Model file for the job. Use its own axes, mm. A direction names the side the tool comes from. Round coordinates to 2 decimals unless told otherwise and drop trailing zeros. Order: outer loops, then holes, each group sorted by start corner. A loop starts at its lowest first (then second) coordinate and runs counter-clockwise, first axis right, second up. Notation, with made-up numbers: (37, 87.25) - (88, 87.25) arc R24 ccw to (88, 123.25) - close; hole circle Ø3 at (2, 13). An arc over 180 degrees is marked (long way). Put each result on its own line as item: value. Start each with the question number.
Item 1: Mould opens along X. For faces 3 (the face through (-285, 10, 5)), 4 (the face through (285, 10, 2)), 5 (the face through (-4, 3, -5)) say: pulls with the +X half, pulls with the -X half, needs draft (parallel to the pull), parting line crosses it, or undercut.
Item 2: Saw through at A-A on x = -91. List the corners of the cut face in (y, z), plus the area to 3 significant figures.
Item 3: Saw through at B-B on z = 13. List the corners of the cut face in (x, y).
Item 4: Probe probe 1 along Y at (x, z) = (25, -1.85); probe 2 along Y at (x, z) = (-11, 15.5); probe 3 along Z at (x, y) = (-195, 5.25). List the from-to ranges inside material, lowest first.
Item 5: Which spindle directions (+Z, -Z, +X, -X, +Y, -Y) get a long thin tool onto all of the face, cutting with end or side? Do faces 1 (the face through (-4, 8, 10)), 2 (the face through (-4, 13, 8)). Say none if no direction does.
```python
from build123d import *

# Parameters (mm, degrees)
F0_W     = 570
F0_H     = 5
F1_DEPTH = 20
F0_R     = 3
F0_W_2   = 5.1
F0_H_2   = 10.1
F0_W_3   = 6
F0_H_3   = 2
F2_DEPTH = 5


with BuildPart() as f1:
    # F0 (on Top) → F1 (new body)
    with BuildSketch(Plane.XY):
        with Locations((0, 10.5)):
            Rectangle(F0_W, F0_H)
    extrude(amount=F1_DEPTH)

    # F0 (on Top) → F2 (join)
    with BuildSketch(Plane.XY):
        with BuildLine():
            ThreePointArc((-285, -5), (-284.12132, -7.12132), (-282, -8))
            Line((-282, -8), (282, -8))
            ThreePointArc((282, -8), (284.12132, -7.12132), (285, -5))
            Line((285, -5), (285, 8))
            Line((285, 8), (-285, 8))
            Line((-285, 8), (-285, -5))
        make_face()
        with Locations((-275, 0)):
            Circle(F0_R, mode=Mode.SUBTRACT)
        with Locations((-220, 0)):
            Circle(F0_R, mode=Mode.SUBTRACT)
        with Locations((-80, 0)):
            Circle(F0_R, mode=Mode.SUBTRACT)
        with Locations((-25, 0)):
            Circle(F0_R, mode=Mode.SUBTRACT)
        Rectangle(F0_W_2, F0_H_2, mode=Mode.SUBTRACT)
        with Locations((25, 0)):
            Circle(F0_R, mode=Mode.SUBTRACT)
        with Locations((80, 0)):
            Circle(F0_R, mode=Mode.SUBTRACT)
        with Locations((220, 0)):
            Circle(F0_R, mode=Mode.SUBTRACT)
        with Locations((275, 0)):
            Circle(F0_R, mode=Mode.SUBTRACT)
        with Locations((-265, 6)):
            Rectangle(F0_W_3, F0_H_3, mode=Mode.SUBTRACT)
        with Locations((-210, 6)):
            Rectangle(F0_W_3, F0_H_3, mode=Mode.SUBTRACT)
        with Locations((-70, 6)):
            Rectangle(F0_W_3, F0_H_3, mode=Mode.SUBTRACT)
        with Locations((-35, 6)):
            Rectangle(F0_W_3, F0_H_3, mode=Mode.SUBTRACT)
        with Locations((35, 6)):
            Rectangle(F0_W_3, F0_H_3, mode=Mode.SUBTRACT)
        with Locations((70, 6)):
            Rectangle(F0_W_3, F0_H_3, mode=Mode.SUBTRACT)
        with Locations((210, 6)):
            Rectangle(F0_W_3, F0_H_3, mode=Mode.SUBTRACT)
        with Locations((265, 6)):
            Rectangle(F0_W_3, F0_H_3, mode=Mode.SUBTRACT)
        with Locations((0, 10.5)):
            Rectangle(F0_W, F0_H)
    extrude(amount=-F2_DEPTH)


solid = f1.part
```
Results found:
1. face 3: pulls with the -X half
1. face 4: pulls with the +X half
1. face 5: needs draft
2. outline: (-8, -5) - (13, -5) - (13, 20) - (8, 20) - (8, 0) - (-8, 0) - close
2. area: 205 mm²
3. outline: (-285, 8) - (285, 8) - (285, 13) - (-285, 13) - close
4. probe 1: y = -8 to -3, 3 to 13
4. probe 2: y = 8 to 13
4. probe 3: z = -5 to 0
5. face 1: +Z, +X, -X, -Y
5. face 2: +Z, -Z, +X, -X, +Y
